For this review, take the finished solid that the model builds, in its own axes (mm). A direction names the side the tool comes from. Round coordinates to 2 decimals unless told otherwise and drop trailing zeros. Order: outer loops, then holes, each group sorted by start corner. A loop starts at its lowest first (then second) coordinate and runs counter-clockwise, first axis right, second up. Notation, with made-up numbers: (22, 56) - (52, 56) arc R20 cw to (52, 66) - close; hole circle Ø6 at (59.5, 6.5). An arc over 180 degrees is marked (long way). Write each question's results on one line, items separated by ' | '. Start each with the question number.
(1) Take a section at C-C, the plane z = 1.9. Give the boundary of the cut face in (x, y).
(2) Take a section at D-D, the plane y = 1.5. Give the boundary of the cut face in (x, z) (3 decimals), plus the area to 3 significant figures.
(3) Take a section at A-A, the plane x = -17. Give the boundary of the cut face in (y, z) (3 decimals), plus the area to 3 significant figures.
(4) For L1, parallel to Y at x = 1, z = 2.65; L2, parallel to Y at x = 12, z = 1.9; L3, parallel to X at y = 6.25, z = 2.5, list the stretches that pass through material, from the lowest coordinate up. Write a range as from..to.
(5) Draft analysis for pull direction Y (two halves, no side actions). For faces 4 (the cylindrical face through (-24.46, -14.61, 1.57)), 5 (the cylindrical face through (15.919, -9.605, 1.565)), 6 (the flat face through (24, 4.238, 2)), state which applies: pulls with the +Y half, pulls with the -Y half, needs draft (parallel to the pull), parting line crosses it, or undercut.
(6) Take a section at B-B, the plane y = -10. Give the boundary of the cut face in (x, z) (3 decimals).
(7) Insertion check: pin 1 Ø1.6 at (y, z) = (6, 1.5) entering from -X; pin 2 Ø1.6 at (x, z) = (23.5, 1.5) entering from +Y; pin 3 Ø1 at (y, z) = (5.5, 2.5) entering from +X; pin 4 Ø1 at (x, y) = (-10, 4.5) entering from -Z. Each pin has a flat end and moves straight along its axis. Give the tip position at first contact, or say it passes through.
(8) For faces 1 (the cylindrical face through (-20.847, -9.655, 1.565)), 2 (the flat face through (21.69, 6, 2)), 3 (the flat face through (-2, 4.238, 2)), list the 3-axis set-ups (+Z, -Z, +X, -X, +Y, -Y) from which the entire face can be reached by the end or side of a thin tool; tool diameter is ignored.
```python
from build123d import *

# Parameters (mm, degrees)
F1_DEPTH = 3.175


with BuildPart() as f1:
    # F0 (on Top) → F1 (new body)
    with BuildSketch(Plane.XY):
        with BuildLine():
            Line((27.01547, 4.237531), (21.689913, 4.237531))
            Line((21.689913, 4.237531), (21.689913, 7.412531))
            Line((21.689913, 7.412531), (11.689913, 7.412531))
            Line((11.689913, 7.412531), (11.689913, 4.237531))
            Line((11.689913, 4.237531), (-16.491257, 4.237531))
            Line((-16.491257, 4.237531), (-16.491257, 7.412531))
            Line((-16.491257, 7.412531), (-26.491257, 7.412531))
            Line((-26.491257, 7.412531), (-26.491257, 4.237531))
            Line((-26.491257, 4.237531), (-32.01359, 4.237531))
            Line((-32.01359, 4.237531), (-26.255299, -12.204799))
            ThreePointArc((-26.255299, -12.204799), (-24.429136, -14.630345), (-21.536318, -15.552159))
            Line((-21.536318, -15.552159), (16.538198, -15.552159))
            ThreePointArc((16.538198, -15.552159), (19.431017, -14.630345), (21.257179, -12.204799))
            Line((21.257179, -12.204799), (27.01547, 4.237531))
        make_face()
        with BuildLine():
            ThreePointArc((17.710482, -7.204799), (15.884319, -9.630345), (12.991501, -10.552159))
            Line((12.991501, -10.552159), (-17.989621, -10.552159))
            ThreePointArc((-17.989621, -10.552159), (-20.882439, -9.630345), (-22.708601, -7.204799))
            Line((-22.708601, -7.204799), (-24.242376, -2.825232))
            ThreePointArc((-24.242376, -2.825232), (-24.043687, -1.415837), (-22.779177, -0.76247))
            Line((-22.779177, -0.76247), (-7.49906, -0.76247))
            Line((-7.49906, -0.76247), (2.50094, -0.76247))
            Line((2.50094, -0.76247), (17.781058, -0.76247))
            ThreePointArc((17.781058, -0.76247), (19.045567, -1.415837), (19.244256, -2.825232))
            Line((19.244256, -2.825232), (17.710482, -7.204799))
        make_face(mode=Mode.SUBTRACT)
    extrude(amount=F1_DEPTH)


solid = f1.part
```
Results below:
1) outline: (-32.01, 4.24) - (-26.26, -12.2) arc R5 ccw to (-21.54, -15.55) - (16.54, -15.55) arc R5 ccw to (21.26, -12.2) - (27.02, 4.24) - (21.69, 4.24) - (21.69, 7.41) - (11.69, 7.41) - (11.69, 4.24) - (-16.49, 4.24) - (-16.49, 7.41) - (-26.49, 7.41) - (-26.49, 4.24) - close; hole (-24.24, -2.83) - (-22.71, -7.2) arc R5 ccw to (-17.99, -10.55) - (12.99, -10.55) arc R5 ccw to (17.71, -7.2) - (19.24, -2.83) arc R1.55 ccw to (17.78, -0.76) - (-22.78, -0.76) arc R1.55 ccw to start
2) outline: (-31.055, 0) - (26.057, 0) - (26.057, 3.175) - (-31.055, 3.175) - close | area: 181 mm^2
3) outline: (-15.552, 0) - (-10.552, 0) - (-10.552, 3.175) - (-15.552, 3.175) - close; (-0.762, 0) - (7.413, 0) - (7.413, 3.175) - (-0.762, 3.175) - close | area: 41.8 mm^2
4) L1: y = -15.55..-10.55, -0.76..4.24 | L2: y = -15.55..-10.55, -0.76..7.41 | L3: x = -26.49..-16.49, 11.69..21.69
5) face 4: pulls with the -Y half | face 5: undercut | face 6: pulls with the +Y half
6) outline: (-27.027, 0) - (-20.274, 0) - (-20.274, 3.175) - (-27.027, 3.175) - close; (15.276, 0) - (22.029, 0) - (22.029, 3.175) - (15.276, 3.175) - close
7) pin 1: stops at x = -26.49 | pin 2: stops at y = 4.24 | pin 3: stops at x = 21.69 | pin 4: stops at z = 0
8) face 1: +Z, -Z | face 2: +Z, -Z, +X, +Y | face 3: +Z, -Z, +Y
